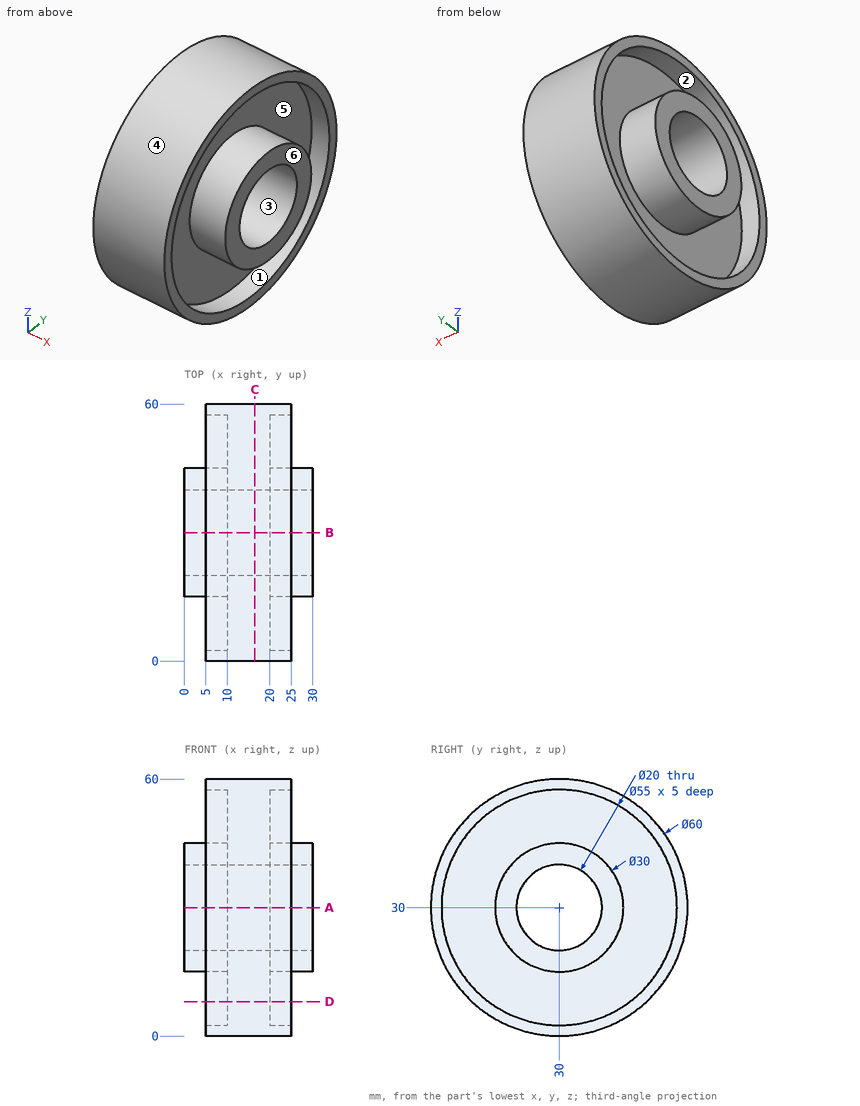
Source: three-view drawing plus pictorial views. Frame: mm from the lowest corner of the part. A direction names the side the tool comes from. Round coordinates to 2 decimals unless told otherwise and drop trailing zeros. Write each loop counter-clockwise with the first axis right and the second up, starting at its lowest first coordinate (ties: lowest second). Pieces come first, ordered by that corner, then holes. Notation, with made-up numbers: M 88,0.5 L 100,0.5 A8 cw 100,9.5 Z; hole C 13.25,-8 d11. An arc over 180 degrees is marked long. Use CSV: the item, a comma, the result in double quotes. Start each with the question number.
Q1. Access query for the marked faces 1, 2 and 3. Directions: +Z, -Z, +X, -X, +Y, -Y. A direction counts if a zero-diameter tool reaches every point of the face in a straight line with its end or side. Return the directions, or none.
Q2. Pull-direction query (Z, two-part tool) for the marked faces 4, 5 and 6; classes: +Z half, -Z half, draft (parallel to the pull), parting line (faces both ways), or undercut.
Q3. Cut plane A-A on z = 30. Output: boundary loops of the cut face in (x, y), plus the area to 3 significant figures.
Q4. Cut plane C-C on x = 16.5. Output: boundary loops of the cut face in (y, z), plus the area to 3 significant figures.
Q5. Line query: line 1 (Z direction, x = 8.3, y = 30); line 2 (Z direction, x = 7.75, y = 25); line 3 (Y direction, x = 23.5, z = 34). Output: solid intervals per line, ascending. Write a range as from..to.
Q6. First-contact query: P1, Ø6, axis at x = 12.5, z = 19.5, coming from the -Y side; P2, Ø1.5, axis at x = 20.5, z = 26, coming from the -Y side; P3, Ø6, axis at x = 16.5, z = 9, coming from the -Y side; P4, Ø18, axis at y = 20.5, z = 31, coming from the -X side. Flat tips, straight axial feed; report the tip coordinate or a pass-through.
Q7. Cut plane D-D on z = 8. Output: boundary loops of the cut face in (x, y).
Results found:
1,face 1,"+X"
1,face 2,"-X"
1,face 3,"+X, -X"
2,face 4,"parting line"
2,face 5,"undercut"
2,face 6,"draft"
3,outline,"M 0,15 L 10,15 L 10,2.5 L 5,2.5 L 5,0 L 25,0 L 25,2.5 L 20,2.5 L 20,15 L 30,15 L 30,20 L 0,20 Z; M 0,40 L 30,40 L 30,45 L 20,45 L 20,57.5 L 25,57.5 L 25,60 L 5,60 L 5,57.5 L 10,57.5 L 10,45 L 0,45 Z"
3,area,"650 mm^2"
4,outline,"C 30,30 d60; hole C 30,30 d20"
4,area,"2,510 mm^2"
5,line 1,"0..2.5, 15..20, 40..45, 57.5..60"
5,line 2,"0.42..2.96, 15.86..21.34, 38.66..44.14, 57.04..59.58"
5,line 3,"0.27..2.79, 15.54..20.83, 39.17..44.46, 57.21..59.73"
6,P1,"y = 0.95"
6,P2,"y = 0.18"
6,P3,"y = 6"
6,P4,"x = 0"
7,outline,"M 5,9.6 L 25,9.6 L 25,13.5 L 20,13.5 L 20,46.5 L 25,46.5 L 25,50.4 L 5,50.4 L 5,46.5 L 10,46.5 L 10,13.5 L 5,13.5 Z"
